```python
from build123d import *

# Parameters (mm, degrees)
BOSS_EXTRUDE1_DEPTH                       = 7.5
CUT_EXTRUDE1_START                        = -10
CUT_EXTRUDE1_DEPTH                        = 5.7
SKETCH5_W                                 = 3.373501
SKETCH5_H                                 = 31.997045256
CUT_EXTRUDE2_START                        = -15
CUT_EXTRUDE2_DEPTH                        = 6
SKETCH8_W                                 = 3.373501
SKETCH8_H                                 = 15
F_17_64_0_26563_DIAMETER_HOLE2_AT_2_COUNT = 2
F_17_64_0_26563_DIAMETER_HOLE2_AT_2_PITCH = 25.4
CUT_EXTRUDE4_START                        = -31
SKETCH10_R                                = 3.373501
CUT_EXTRUDE4_DEPTH                        = 31
CUT_EXTRUDE5_START                        = -25.7
SKETCH11_R                                = 3.373501
CUT_EXTRUDE5_DEPTH                        = 25.7


with BuildPart() as part:
    # Sketch1 → Boss-Extrude1 (new, symmetric)
    with BuildSketch(Plane.XY):
        Polygon((0, -28.802954744), (0, 28.802954744), (-25.4, 72.797045256), (-50.8, 72.797045256), (-50.8, -28.802954744), (-25.4, -28.802954744), align=None)
    extrude(amount=BOSS_EXTRUDE1_DEPTH, both=True)

    # Sketch2 → Cut-Extrude1 (cut)
    with BuildSketch(Plane(origin=(12.472045256, 7.200738686, 0), x_dir=(0, 0, -1), z_dir=(0.8660254037844379, 0.5000000000000013, 0)).offset(CUT_EXTRUDE1_START)):
        Polygon((3.464101615, 33.944090512), (7.5, 33.944090512), (7.5, 45.944090512), (3.464101615, 45.944090512), (-3.464101615, 45.944090512), (-7.5, 45.944090512), (-7.5, 33.944090512), (-3.464101615, 33.944090512), align=None)
    extrude(amount=-CUT_EXTRUDE1_DEPTH, mode=Mode.SUBTRACT)

    # Sketch5 → 17/64 (0.26563) Diameter Hole1 (revolve, cut)
    with BuildSketch(Plane(origin=(-16.160254038, 36.793335801, 0), x_dir=(0.500000000000001, -0.866025403784438, 0), z_dir=(0, 0, 1))):
        with Locations((1.6867505, 15.998522628)):
            Rectangle(SKETCH5_W, SKETCH5_H)
    revolve(axis=Axis((-21.659515352, 33.618335801, 0), (0.866025403784438, 0.500000000000001, 0)), mode=Mode.SUBTRACT)

    # Sketch6 → Cut-Extrude2 (cut)
    with BuildSketch(Plane.XZ.offset(28.802954744).offset(CUT_EXTRUDE2_START)):
        Polygon((-43.95, 3.377499075), (-43.95, -3.377499075), (-43.95, -7.5), (-32.25, -7.5), (-32.25, -3.377499075), (-32.25, 3.377499075), (-32.25, 7.5), (-43.95, 7.5), align=None)
        Polygon((-18.55, 3.377499075), (-18.55, -3.377499075), (-18.55, -7.5), (-6.85, -7.5), (-6.85, -3.377499075), (-6.85, 3.377499075), (-6.85, 7.5), (-18.55, 7.5), align=None)
    extrude(amount=-CUT_EXTRUDE2_DEPTH, mode=Mode.SUBTRACT)

    # Sketch8 → 17/64 (0.26563) Diameter Hole2 (revolve, cut)
    with BuildSketch(Plane(origin=(-38.1, -13.802954744, 0), x_dir=(0, 0, 1), z_dir=(1, 0, 0))):
        with Locations((1.6867505, 7.5)):
            Rectangle(SKETCH8_W, SKETCH8_H)
    f_17_64_0_26563_diameter_hole2 = revolve(axis=Axis((-38.1, -7.452954744, 0), (0, -1, 0)), mode=Mode.SUBTRACT)

    # 17/64 (0.26563) Diameter Hole2 at 2: 17/64 (0.26563) Diameter Hole2 ×2
    with Locations(*[(i * F_17_64_0_26563_DIAMETER_HOLE2_AT_2_PITCH, 0, 0) for i in range(1, F_17_64_0_26563_DIAMETER_HOLE2_AT_2_COUNT)]):
        add(f_17_64_0_26563_diameter_hole2, mode=Mode.SUBTRACT)

    # Sketch10 → Cut-Extrude4 (cut)
    with BuildSketch(Plane.XZ.offset(28.802954744).offset(CUT_EXTRUDE4_START)):
        with Locations(Location((-38.1, 0, 0), (0, 0, 90))):
            Circle(SKETCH10_R)
        with Locations(Location((-12.7, 0, 0), (0, 0, 90))):
            Circle(SKETCH10_R)
    extrude(amount=CUT_EXTRUDE4_DEPTH, mode=Mode.SUBTRACT)

    # Sketch11 → Cut-Extrude5 (cut)
    with BuildSketch(Plane(origin=(12.472045256, 7.200738686, 0), x_dir=(0, 0, -1), z_dir=(0.8660254037844378, 0.5000000000000017, 0)).offset(CUT_EXTRUDE5_START)):
        with Locations(Location((0, 39.944090512, 0), (0, 0, 270))):
            Circle(SKETCH11_R)
    extrude(amount=CUT_EXTRUDE5_DEPTH, mode=Mode.SUBTRACT)


solid = part.part
```
Input: part model. Units: mm. Frame: model coordinates. A direction names the side the tool comes from. Give positions to 0.01 mm unless a question says otherwise; leave off trailing zeros. Loops run counter-clockwise (first coordinate to the right, second up) from the corner with the lowest first, then second, coordinate; pieces in that order, holes last. Notation, with made-up numbers: M 87,13.25 L 99,13.25 A16 ccw 99,36.25 Z; hole C 6.25,-18.75 d2. An arc over 180 degrees is marked long. Answer as CSV lines item,"result". Start each with the question number.
1. Line query: L1, parallel to X at y = -24.25, z = 0; L2, parallel to X at y = -10.5, z = -4; L3, parallel to Z at x = -38.1, y = -1. Output: solid intervals per line, ascending.
2. Pull-direction query (Y, two-part tool) for faces 5 (the face through (-21.594, 40.584, -0.105)), 6 (the face through (-13, 2.197, 0)), 7 (the face through (-9.4, -2.7, -0.7)); classes: released by +Y, released by -Y, zero draft, split by the parting line, or undercut.
3. Section A-A on x = -38.1. Return loops of the section in (y, z).
4. Section C-C on y = 49. Return loops of the section in (x, z), plus the area to 3 significant figures.
5. Section D-D on x = -3.5. Return loops of the section in (y, z).
6. Section B-B on z = -5.75. Return loops of the section in (x, y).
7. Pin query (flat end, axial travel): P1, Ø6, axis at x = -38.1, z = 0, coming from the -Y side; P2, Ø4, axis at x = -12.7, z = 0, coming from the +Y side; P3, Ø3.5, axis at x = -14.5, z = -1, coming from the +Y side. Return the tip coordinate at first contact, or that it passes through.
8. Reachability of faces 1 (the face through (-18.55, -11, 0)), 2 (the face through (-29.78, 28.98, -0.05)), 3 (the face through (-26, -28.803, 0)), 4 (the face through (-38, 2.197, 0)) from +Z, -Z, +X, -X, +Y, -Y: full face, straight path, thin tool, end or side. Return the list, or none.
Computed values:
1,L1,"x = -50.8 to -41.47, -34.73 to -16.07, -9.33 to 0"
1,L2,"x = -50.8 to -43.95, -32.25 to -18.55, -6.85 to 0"
1,L3,"z = -7.5 to -3.37, 3.37 to 7.5"
2,face 5,"undercut"
2,face 6,"released by -Y"
2,face 7,"zero draft"
3,outline,"M -28.8,-7.5 L -13.8,-7.5 L -13.8,-3.37 L -28.8,-3.37 Z; M -28.8,3.37 L -13.8,3.37 L -13.8,7.5 L -28.8,7.5 Z; M -7.8,-7.5 L 72.8,-7.5 L 72.8,7.5 L -7.8,7.5 L -7.8,3.37 L 2.2,3.37 L 2.2,-3.37 L -7.8,-3.37 Z"
4,outline,"M -50.8,-7.5 L -11.66,-7.5 L -11.66,7.5 L -50.8,7.5 Z"
4,area,"587 mm²"
5,outline,"M -28.8,-7.5 L 34.87,-7.5 L 34.87,7.5 L -28.8,7.5 Z"
6,outline,"M -50.8,-28.8 L 0,-28.8 L 0,28.8 L -25.4,72.8 L -50.8,72.8 Z; hole M -43.95,-13.8 L -32.25,-13.8 L -32.25,-7.8 L -43.95,-7.8 Z; hole M -24.1,39.14 L -18.1,28.75 L -13.16,31.6 L -19.16,41.99 Z; hole M -18.55,-13.8 L -6.85,-13.8 L -6.85,-7.8 L -18.55,-7.8 Z"
7,P1,"stops at y = 2.2"
7,P2,"stops at y = 54.26"
7,P3,"stops at y = 56.95"
8,face 1,"+Z, -Z"
8,face 2,"none"
8,face 3,"+Z, -Z, +X, -X, -Y"
8,face 4,"-Y"
